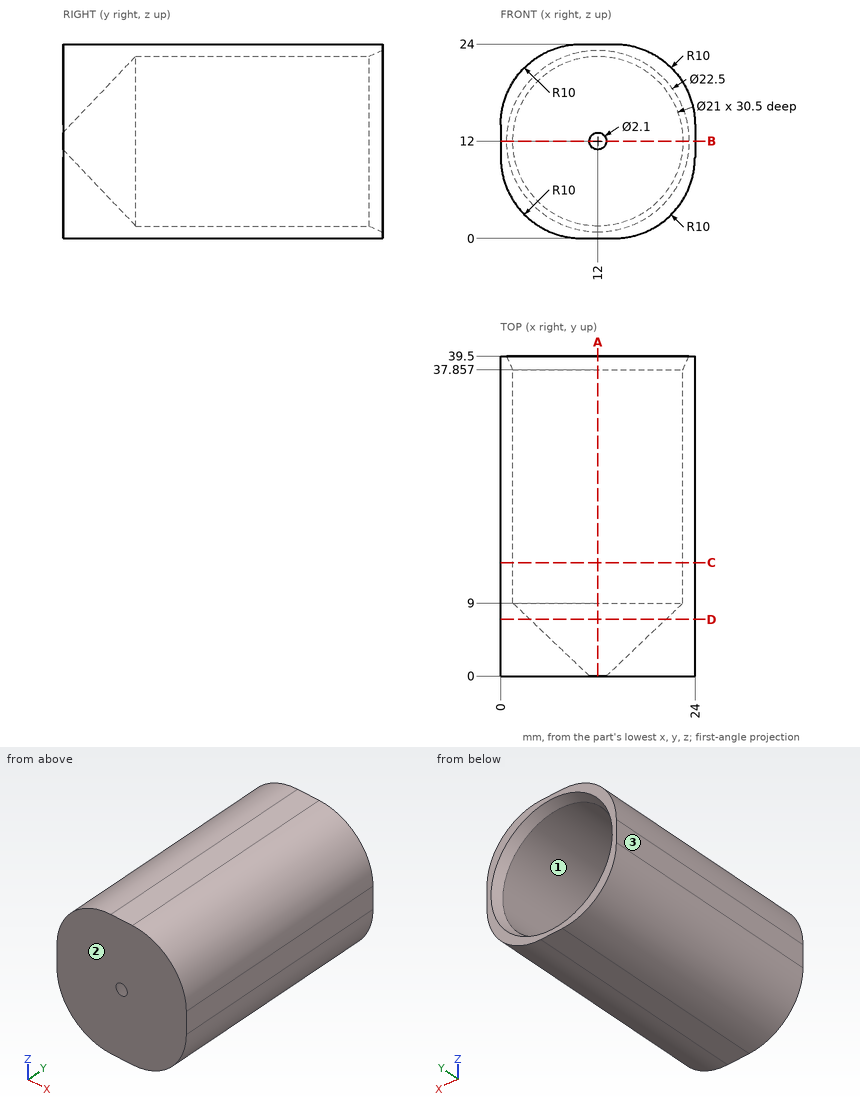
Input: dimensioned drawing with shaded views. Units: mm. Origin: part minimum x, y, z. Give positions to 0.01 mm unless a question says otherwise; leave off trailing zeros. Write each loop counter-clockwise with the first axis right and the second up, starting at its lowest first coordinate (ties: lowest second). Pieces come first, ordered by that corner, then holes.
1. Section query A-A, the plane x = 12. Return loops of the section in (y, z).
2. Section query B-B, the plane z = 12. Return loops of the section in (x, y).
3. Line query: probe 1 along X at (y, z) = (26.75, 12); probe 2 along X at (y, z) = (25.5, 20.5) (1 decimal); probe 3 along Z at (x, y) = (9.75, 20). Output: solid intervals per line, ascending.
4. Section query C-C, the plane y = 14. Return loops of the section in (x, z), then the cut area to 3 significant figures.
5. Draft query along X for the marked faces 1, 2 and 3. Return one class per face: released by +X, released by -X, zero draft, split by the parting line, or undercut.
6. Section query D-D, the plane y = 7. Return loops of the section in (x, z).
7. Pin query (flat end, axial travel): P1, Ø2, axis at x = 12.5, z = 18.5, coming from the +Y side; P2, Ø6, axis at x = 17.5, y = 28, coming from the +Z side; P3, Ø10, axis at y = 31, z = 3.5, coming from the -X side. Return the tip coordinate at first contact, or that it passes through.
Computed:
1. outline: (0, 0) - (39.5, 0) - (39.5, 0.75) - (37.86, 1.5) - (9, 1.5) - (0, 10.95) - close; (0, 13.05) - (9, 22.5) - (37.86, 22.5) - (39.5, 23.25) - (39.5, 24) - (0, 24) - close
2. outline: (0, 0) - (10.95, 0) - (1.5, 9) - (1.5, 37.86) - (0.75, 39.5) - (0, 39.5) - close; (13.05, 0) - (24, 0) - (24, 39.5) - (23.25, 39.5) - (22.5, 37.86) - (22.5, 9) - close
3. probe 1: x = 0 to 1.5, 22.5 to 24
3. probe 2: x = 2.4 to 5.8, 18.2 to 21.6
3. probe 3: z = 0 to 1.74, 22.26 to 24
4. outline: (0, 10) arc R10 ccw to (10, 0) - (14, 0) arc R10 ccw to (24, 10) - (24, 14) arc R10 ccw to (14, 24) - (10, 24) arc R10 ccw to (0, 14) - close; hole circle Ø21 at (12, 12)
4. area: 144 mm2
5. face 1: undercut
5. face 2: zero draft
5. face 3: released by -X
6. outline: (0, 10) arc R10 ccw to (10, 0) - (14, 0) arc R10 ccw to (24, 10) - (24, 14) arc R10 ccw to (14, 24) - (10, 24) arc R10 ccw to (0, 14) - close; hole circle Ø16.8 at (12, 12)
7. P1: stops at y = 6.16
7. P2: stops at z = 23.99
7. P3: stops at x = 0.11
